Solid Edge part; units mm, degrees
sketch "Sketch1" plane through (0, 0, 0) normal (0, 0, 1) x (1, 0, 0)
  line L0 (0, 0) -> (0, 263.525)
sketch "Sketch2" plane through (0, 0, 0) normal (0, -1, 0) x (1, 0, 0)
  line L0 (4.572, 12.7) -> (-4.572, 12.7)
  arc A0 (-4.572, 12.7) -> (-6.35, 10.922) centre (-4.572, 10.922) ccw
  line L1 (-6.35, 10.922) -> (-6.35, -10.922)
  arc A1 (-4.572, -12.7) -> (-6.35, -10.922) centre (-4.572, -10.922) cw
  line L2 (-4.572, -12.7) -> (4.572, -12.7)
  arc A2 (4.572, -12.7) -> (6.35, -10.922) centre (4.572, -10.922) ccw
  line L3 (6.35, -10.922) -> (6.35, 10.922)
  arc A3 (6.35, 10.922) -> (4.572, 12.7) centre (4.572, 10.922) ccw
sweep "SweptProtrusion1" add profiles "Sketch2" path "Sketch1"
sketch "Sketch3" plane through (0, 0, 0) normal (0, 0, 1) x (1, 0, 0)
  line L0 (0, 0) -> (0, 263.525)
sketch "Sketch4" plane through (-6.35, 0, 6.35) normal (0, -1, 0) x (1, 0, 0)
  circle A0 centre (3.9624, 2.3876) radius 2.032
sweep "SweptCutout1" cut profiles "Sketch4" path "Sketch3"
sketch "Sketch5" plane through (0, 0, 0) normal (0, 0, 1) x (1, 0, 0)
  line L0 (0, 0) -> (0, 263.525)
sketch "Sketch6" plane through (-6.35, 0, 6.35) normal (0, -1, 0) x (1, 0, 0)
  circle A0 centre (3.9624, -15.0876) radius 2.032
sweep "SweptCutout2" cut profiles "Sketch6" path "Sketch5"
sketch "Sketch7" plane through (0, 0, 0) normal (0, 0, 1) x (1, 0, 0)
  line L0 (0, 0) -> (0, 263.525)
sketch "Sketch8" plane through (0, 0, 0) normal (0, -1, 0) x (1, 0, 0)
  line L0 (4.1402, 3.7973) -> (4.1402, 5.2661)
  arc A0 (4.1402, 5.2661) -> (2.2806, 6.2777) centre (2.9353, 5.2661) ccw
  line L1 (-3.147, 2.7652) -> (2.2806, 6.2777)
  arc A1 (-3.495, 2.1255) -> (-3.147, 2.7652) centre (-2.733, 2.1255) cw
  line L2 (-3.495, 2.1255) -> (-3.495, -2.1255)
  arc A2 (-3.495, -2.1255) -> (-3.147, -2.7652) centre (-2.733, -2.1255) ccw
  line L3 (-3.147, -2.7652) -> (2.2806, -6.2777)
  arc A3 (4.1402, -5.2661) -> (2.2806, -6.2777) centre (2.9353, -5.2661) cw
  line L4 (4.1402, -3.7846) -> (4.1402, -5.2661)
  line L5 (6.35, 3.7973) -> (6.35, -3.7846)
  arc A4 (4.1402, -3.7846) -> (6.35, -3.7846) centre (5.2451, -3.7846) cw
  arc A5 (6.35, 3.7973) -> (4.1402, 3.7973) centre (5.2451, 3.7973) cw
sweep "SweptCutout3" cut profiles "Sketch8" path "Sketch7"
sketch "Sketch9" plane through (0, 0, 0) normal (0, 0, 1) x (1, 0, 0)
  line L0 (0, 0) -> (0, 263.525)
sketch "Sketch10" plane through (0, 0, 0) normal (0, -1, 0) x (-1, 0, 0)
  circle A0 centre (6.35, -10.795) radius 0.381
sweep "SweptCutout4" cut profiles "Sketch10" path "Sketch9"
sketch "Sketch11" plane through (0, 0, 0) normal (0, 0, 1) x (1, 0, 0)
  line L0 (0, 0) -> (0, 263.525)
sketch "Sketch12" plane through (0, 0, 0) normal (0, -1, 0) x (0, 0, 1)
  circle A0 centre (7.366, 6.35) radius 0.381
sweep "SweptCutout5" cut profiles "Sketch12" path "Sketch11"
sketch "Sketch13" plane through (0, 0, 0) normal (0, 0, 1) x (1, 0, 0)
  line L0 (0, 0) -> (0, 263.525)
sketch "Sketch14" plane through (0, 0, 0) normal (0, -1, 0) x (-1, 0, 0)
  circle A0 centre (-6.35, -10.795) radius 0.381
sweep "SweptCutout6" cut profiles "Sketch14" path "Sketch13"
sketch "Sketch15" plane through (0, 0, 0) normal (0, 0, 1) x (1, 0, 0)
  line L0 (0, 0) -> (0, 263.525)
sketch "Sketch16" plane through (0, 0, 0) normal (0, -1, 0) x (0, 0, 1)
  circle A0 centre (7.3678, -6.35) radius 0.381
sweep "SweptCutout7" cut profiles "Sketch16" path "Sketch15"
sketch "Sketch17" plane through (0, 0, 0) normal (0, 0, 1) x (1, 0, 0)
  line L0 (0, 0) -> (0, 263.525)
sketch "Sketch18" plane through (0, 0, 0) normal (0, -1, 0) x (0, 0, -1)
  circle A0 centre (10.795, -6.35) radius 0.381
sweep "SweptCutout8" cut profiles "Sketch18" path "Sketch17"
sketch "Sketch19" plane through (0, 0, 0) normal (0, 0, 1) x (1, 0, 0)
  line L0 (0, 0) -> (0, 263.525)
sketch "Sketch20" plane through (0.0001, 0, 0) normal (0, -1, 0) x (0, 0, -1)
  circle A0 centre (6.985, -6.3501) radius 0.381
sweep "SweptCutout9" cut profiles "Sketch20" path "Sketch19"
sketch "Sketch21" plane through (0, 0, 0) normal (0, 0, 1) x (1, 0, 0)
  line L0 (0, 0) -> (0, 263.525)
sketch "Sketch22" plane through (0.0001, 0, 0) normal (0, -1, 0) x (0, 0, -1)
  circle A0 centre (10.795, 6.3499) radius 0.381
sweep "SweptCutout10" cut profiles "Sketch22" path "Sketch21"
sketch "Sketch23" plane through (0, 0, 0) normal (0, 0, 1) x (1, 0, 0)
  line L0 (0, 0) -> (0, 263.525)
sketch "Sketch24" plane through (0.0001, 0, 0) normal (0, -1, 0) x (0, 0, 1)
  circle A0 centre (-7.0993, -6.3499) radius 0.3937
sweep "SweptCutout11" cut profiles "Sketch24" path "Sketch23"
Input: part model. Units: mm. Frame: model coordinates. A direction names the side the tool comes from. Coordinates: 2 decimals unless noted, no trailing zeros.
(1) Pull-direction query (X, two-part tool) for faces 3 (the face through (-3.495, 134, 0)), 4 (the face through (-2.83, 133.61, 10.72)), 5 (the face through (-4, 0, 0)); classes: released by +X, released by -X, zero draft, split by the parting line, or undercut.
(2) First-contact query: pin 1 Ø1.5 at (y, z) = (153, -1) entering from +X (3 decimals). Flat tip, straight axial feed; report the tip coordinate or a pass-through.
(3) Set-up query: faces 1 (the face through (-0.395, 133.607, 4.546)), 2 (the face through (0, 134, 12.7)). Return all of +Z, -Z, +X, -X, +Y, -Y with unobstructed straight access to the full face (end or side cutting, diameter ignored); none if empty.
(4) Material intervals for probe 1 along Z at (x, y) = (3.5, 181); probe 2 along Z at (x, y) = (-3.75, 187); probe 3 along Z at (x, y) = (0.75, 121), sorted ascending.
(5) Section A-A on y = 131. Count the separate pieces of the cut face and the enclosed holes in it, then the cut area to 3 significant figures.
Data:
1. face 3: released by +X
1. face 4: undercut
1. face 5: zero draft
2. pin 1: stops at x = -3.495
3. face 1: +Y, -Y
3. face 2: +Z, +X, -X, +Y, -Y
4. probe 1: z = -12.7 to -6.33, 6.33 to 12.7
4. probe 2: z = -12.7 to -10.25, -7.23 to 7.23, 10.25 to 12.7
4. probe 3: z = -12.7 to -5.29, 5.29 to 12.7
5. separate pieces: 1
5. enclosed holes: 2
5. area: 205 mm2
